Can you work these out from the model? Positions are in its coordinate system, mm. A direction names the side the tool comes from. Round coordinates to 2 decimals unless told otherwise and drop trailing zeros. Write each loop counter-clockwise with the first axis right and the second up, starting at its lowest first coordinate (ties: lowest second). Pieces come first, ordered by that corner, then holes. Notation, with made-up numbers: (57.25, -0.75) -> (100.25, -0.75) arc R21 ccw to (100.25, 28.25) -> close; hole circle Ø7 at (42.5, 37.5). An arc over 180 degrees is marked (long way). Write item = value, one per line. Start each with the question number.
1) I'm going to push flat-ended pins straight in: pin 1 (14 mm diameter, centred on y = -0.5, z = 20, fed in from -X); pin 2 (3 mm diameter, centred on x = 0.5, z = 7, fed in from -Y); pin 3 (1.6 mm diameter, centred on x = 0, z = 14, fed in from -Y). Where does each tip first touch, or does it pass through?
2) Thinking about a two-plate mould opening in Y: for faces 1 (the face through (-4.01, -13.057, 2.73)), 2 (the face through (0.04, -16.3, 3.63)), 3 (the face through (-1.588, 0, 18)), which applies, +Y half, -Y half, draft (parallel to the pull), parting line (faces both ways), or undercut?
3) Imagine slicing it at C-C, the plane z = 25.5. Please give me the cut outline in (x, y), then the cut area to 3 significant figures.
4) Imagine slicing it at D-D, the plane y = 9.5. Please give me the cut outline in (x, z) (1 decimal), then the cut area to 3 significant figures.
5) For faces 4 (the face through (4.01, 18.982, 2.717)), 5 (the face through (0, 12.598, 3)), 6 (the face through (4.01, -13.057, 2.73)), 7 (the face through (3.987, -15.43, 8.756)), which set-ups out of +Z, -Z, +X, -X, +Y, -Y let a thin tool reach every point of the face, with its end or its side?
6) Imagine slicing it at A-A, the plane x = -0.25. Please give me the cut outline in (y, z) (3 decimals).
7) Imagine slicing it at B-B, the plane y = 0. Please give me the cut outline in (x, z) (1 decimal), then the cut area to 3 significant figures.
8) If I drill on line 1 (Y direction, x = -1, z = 5); line 2 (X direction, y = -6.5, z = 21); line 3 (Y direction, x = -0.25, z = 19.5), over which ranges is the centre line in solid material (lowest first)?
from build123d import *

# Parameters (mm, degrees)
BOSS_EXTRUDE1_DEPTH = 4.445
BOSS_EXTRUDE2_DEPTH = 1.5875
SKETCH5_R           = 3.81
CUT_EXTRUDE1_DEPTH  = 127
FILLET2_R           = 1.524
FILLET3_R           = 1.524
FILLET4_R           = 1.524


with BuildPart() as part:
    # Sketch3 → Boss-Extrude1 (new, symmetric)
    with BuildSketch(Plane.YZ):
        Polygon((-19.8628, 0), (-19.8628, 3.175), (-15.86484, 3.175), (-15.86484, 12.7), (15.86484, 12.7), (15.86484, 3.175), (21.4122, 3.175), (21.4122, 0), (12.5984, 0), (12.5984, 7.0612), (-12.5984, 7.0612), (-12.5984, 0), align=None)
    extrude(amount=BOSS_EXTRUDE1_DEPTH, both=True)

    # Sketch4 → Boss-Extrude2 (add, symmetric)
    with BuildSketch(Plane.YZ):
        with BuildLine():
            Line((-14.224, 12.7), (-14.224, 15.875))
            ThreePointArc((-14.224, 15.875), (0, 30.099), (14.224, 15.875))
            Line((14.224, 15.875), (14.224, 12.7))
            Line((14.224, 12.7), (15.86484, 12.7))
            Line((15.86484, 12.7), (15.86484, 3.175))
            Line((15.86484, 3.175), (21.4122, 3.175))
            Line((21.4122, 3.175), (21.4122, 0))
            Line((21.4122, 0), (12.5984, 0))
            Line((12.5984, 0), (12.5984, 7.0612))
            Line((12.5984, 7.0612), (-12.5984, 7.0612))
            Line((-12.5984, 7.0612), (-12.5984, 0))
            Line((-12.5984, 0), (-19.8628, 0))
            Line((-19.8628, 0), (-19.8628, 3.175))
            Line((-19.8628, 3.175), (-15.86484, 3.175))
            Line((-15.86484, 3.175), (-15.86484, 12.7))
            Line((-15.86484, 12.7), (-14.224, 12.7))
        make_face()
    extrude(amount=BOSS_EXTRUDE2_DEPTH, both=True)

    # Sketch5 → Cut-Extrude1 (cut)
    with BuildSketch(Plane.YZ.offset(4.445)):
        with Locations(Location((0, 22.873624204, 0), (0, 0, 90))):
            Circle(SKETCH5_R)
    extrude(amount=-CUT_EXTRUDE1_DEPTH, mode=Mode.SUBTRACT)

    # Fillet2
    fillet2_edges = [part.edges().sort_by_distance(p)[0] for p in [
        (4.445, 15.86484, 7.9375),
        (4.445, 18.63852, 3.175),
        (0, 15.86484, 12.7),
        (0, 15.86484, 3.175),
        (0, 21.4122, 3.175),
        (-4.445, 18.63852, 3.175),
        (-4.445, 15.86484, 7.9375),
    ]]
    fillet(fillet2_edges, radius=FILLET2_R)

    # Fillet3
    fillet3_edges = [part.edges().sort_by_distance(p)[0] for p in [
        (4.445, -17.86382, 3.175),
        (4.445, -15.86484, 7.9375),
        (0, -15.86484, 3.175),
        (0, -15.86484, 12.7),
        (-4.445, -15.86484, 7.9375),
        (-4.445, -17.86382, 3.175),
    ]]
    fillet(fillet3_edges, radius=FILLET3_R)

    # Fillet4
    fillet4_edges = [part.edges().sort_by_distance(p)[0] for p in [
        (-4.445, 0, 7.0612),
        (4.445, 12.5984, 3.5306),
        (4.445, 0, 7.0612),
        (4.445, -12.5984, 3.5306),
        (-4.445, 12.5984, 3.5306),
        (0, 12.5984, 7.0612),
        (0, -12.5984, 7.0612),
        (-4.445, -12.5984, 3.5306),
    ]]
    fillet(fillet4_edges, radius=FILLET4_R)


solid = part.part
Reported:
q1.pin_1 = -1.59
q1.pin_2 = -15.86
q1.pin_3 = -14.22
q2.face_1 = undercut
q2.face_2 = -Y half
q2.face_3 = draft
q3.outline = (-1.59, -10.47) -> (1.59, -10.47) -> (1.59, -2.76) -> (-1.59, -2.76) -> close; (-1.59, 2.76) -> (1.59, 2.76) -> (1.59, 10.47) -> (-1.59, 10.47) -> close
q3.area = 49.0 mm²
q4.outline = (-4.4, 8.6) arc R1.5 ccw to (-2.9, 7.1) -> (2.9, 7.1) arc R1.5 ccw to (4.4, 8.6) -> (4.4, 12.7) -> (1.6, 12.7) -> (1.6, 26.5) -> (-1.6, 26.5) -> (-1.6, 12.7) -> (-4.4, 12.7) -> close
q4.area = 92.8 mm²
q5.face_4 = +Z, +X, +Y
q5.face_5 = -Z, +X, -X
q5.face_6 = -Z, +X
q5.face_7 = +Z, +X, -Y
q6.outline = (-19.863, 0) -> (-12.598, 0) -> (-12.598, 5.537) arc R1.524 cw to (-11.074, 7.061) -> (11.074, 7.061) arc R1.524 cw to (12.598, 5.537) -> (12.598, 0) -> (21.412, 0) -> (21.412, 1.651) arc R1.524 ccw to (19.888, 3.175) -> (17.389, 3.175) arc R1.524 cw to (15.865, 4.699) -> (15.865, 11.176) arc R1.524 ccw to (14.341, 12.7) -> (14.224, 12.7) -> (14.224, 15.875) arc R14.224 ccw to (-14.224, 15.875) -> (-14.224, 12.7) -> (-14.341, 12.7) arc R1.524 ccw to (-15.865, 11.176) -> (-15.865, 4.699) arc R1.524 cw to (-17.389, 3.175) -> (-19.863, 3.175) -> close; hole circle Ø7.62 at (0, 22.874)
q7.outline = (-4.4, 8.6) arc R1.5 ccw to (-2.9, 7.1) -> (2.9, 7.1) arc R1.5 ccw to (4.4, 8.6) -> (4.4, 12.7) -> (1.6, 12.7) -> (1.6, 19.1) -> (-1.6, 19.1) -> (-1.6, 12.7) -> (-4.4, 12.7) -> close; (-1.6, 26.7) -> (1.6, 26.7) -> (1.6, 30.1) -> (-1.6, 30.1) -> close
q7.area = 80.2 mm²
q8.line_1 = -15.86 to -12.6, 12.6 to 15.86
q8.line_2 = -1.59 to 1.59
q8.line_3 = -13.75 to -1.77, 1.77 to 13.75
